```python
from build123d import *

# Parameters (mm, degrees)
SKETCH_1_R      = 1.5
SKETCH_1_R_2    = 0.5
SKETCH_1_W      = 23
SKETCH_1_H      = 12
EXTRUDE_1_DEPTH = 3


with BuildPart() as part:
    # 草图1 → 凸台-拉伸1 (new body)
    with BuildSketch(Plane(origin=(0, 0, 0), x_dir=(1, 0, 0), z_dir=(0, 1, 0))):
        Polygon((22.594315567, 25.84326654), (22.594315567, 28.84326654), (-7.405684433, 28.84326654), (-7.405684433, 25.84326654), (-10.405684433, 25.84326654), (-10.405684433, 28.84326654), (-40.405684433, 28.84326654), (-40.405684433, 25.84326654), (-43.405684433, 25.84326654), (-43.405684433, 28.84326654), (-44.905684433, 28.84326654), (-44.905684433, 10.84326654), (-43.405684433, 10.84326654), (-43.405684433, 13.84326654), (-40.405684433, 13.84326654), (-40.405684433, 10.84326654), (-10.405684433, 10.84326654), (-10.405684433, 14.84326654), (-7.405684433, 14.84326654), (-7.405684433, 10.84326654), (22.594315567, 10.84326654), (22.594315567, 13.84326654), (25.594315567, 13.84326654), (25.594315567, 10.84326654), (27.094315567, 10.84326654), (27.094315567, 28.84326654), (25.594315567, 28.84326654), (25.594315567, 25.84326654), align=None)
        with Locations(Location((-8.905684433, 19.84326654, 0), (0, 0, 270))):
            Circle(SKETCH_1_R, mode=Mode.SUBTRACT)
        with Locations(Location((-4.505684433, 19.84326654, 0), (0, 0, 270))):
            Circle(SKETCH_1_R_2, mode=Mode.SUBTRACT)
        with Locations(Location((-40.805684433, 19.84326654, 0), (0, 0, 270))):
            Circle(SKETCH_1_R_2, mode=Mode.SUBTRACT)
        with Locations(Location((-13.305684433, 19.84326654, 0), (0, 0, 270))):
            Circle(SKETCH_1_R_2, mode=Mode.SUBTRACT)
        with Locations(Location((22.994315567, 19.84326654, 0), (0, 0, 270))):
            Circle(SKETCH_1_R_2, mode=Mode.SUBTRACT)
        with Locations((9.094315567, 19.84326654)):
            Rectangle(SKETCH_1_W, SKETCH_1_H, mode=Mode.SUBTRACT)
        with Locations((-26.905684433, 19.84326654)):
            Rectangle(SKETCH_1_W, SKETCH_1_H, mode=Mode.SUBTRACT)
    extrude(amount=EXTRUDE_1_DEPTH)


solid = part.part
```
Work out the finished part from the listing and answer in its coordinate system (mm). A direction names the side the tool comes from. Give positions to 0.01 mm unless a question says otherwise; leave off trailing zeros. Loops run counter-clockwise (first coordinate to the right, second up) from the corner with the lowest first, then second, coordinate; pieces in that order, holes last. Notation, with made-up numbers: (-1.5, 24.25) -> (22.5, 24.25) arc R19 ccw to (22.5, 37.25) -> close; hole circle Ø11 at (-16.5, 14). An arc over 180 degrees is marked (long way). Put each result on its own line as item: value. Start each with the question number.
Item 1: Each of these flat-tipped pins is pushed along its axis until it touches: P1, Ø1.8, axis at x = -8.91, z = -19.84, coming from the +Y side; P2, Ø0.9, axis at x = 24.5, y = 1.5, coming from the +Z side. Where does it stop, or does it pass through?
Item 2: The part is cut by section C-C (z = -26.5). Give the vertices of the cut face in (x, y), then the cut area to 3 significant figures.
Item 3: Which of the six approach directions +Z, -Z, +X, -X, +Y, -Y give full straight-line access (tool end or side, diameter ignored) to faces 4 (the face through (-10.406, 1, -13)), 5 (the face through (-25, 1, -28.843)), 6 (the face through (-15.406, 1, -20)), 7 (the face through (-42, 1, -25.843))?
Item 4: The part is cut by section B-B (z = -16). Give the vertices of the cut face in (x, y), then the cut area to 3 significant figures.
Item 5: Find the intervals of material crossed by L1, parallel to X at y = 2.6, z = -17.5; L2, parallel to X at y = 1.65, z = -27; L3, parallel to X at y = 1.4, z = -14.75, in increasing order. Write a range as [from, to].
Item 6: The mould has two halves that part along X. Classify faces 1 (the face through (-9, 3, -22)), 2 (the face through (-44.906, 1, -20)), 3 (the face through (-42, 1, -13.843)): released by +X, released by -X, zero draft, split by the parting line, or undercut.
Item 7: The part is cut by section A-A (x = -30.5). Give the vertices of the cut face in (y, z).
Item 8: The part is cut by section D-D (y = 0.75). State how many separate pieces and enclosed holes the cut face has, then the cut area to 3 significant figures.
Answers below:
1. P1: through
1. P2: z = -13.84
2. outline: (-44.91, 0) -> (-43.41, 0) -> (-43.41, 3) -> (-44.91, 3) -> close; (-40.41, 0) -> (-10.41, 0) -> (-10.41, 3) -> (-40.41, 3) -> close; (-7.41, 0) -> (22.59, 0) -> (22.59, 3) -> (-7.41, 3) -> close; (25.59, 0) -> (27.09, 0) -> (27.09, 3) -> (25.59, 3) -> close
2. area: 189 mm2
3. face 4: +Z, +Y, -Y
3. face 5: -Z, +X, -X, +Y, -Y
3. face 6: +Y, -Y
3. face 7: -Z, +Y, -Y
4. outline: (-44.91, 0) -> (-38.41, 0) -> (-38.41, 3) -> (-44.91, 3) -> close; (-15.41, 0) -> (-2.41, 0) -> (-2.41, 3) -> (-15.41, 3) -> close; (20.59, 0) -> (27.09, 0) -> (27.09, 3) -> (20.59, 3) -> close
4. area: 78.0 mm2
5. L1: [-44.91, -38.41], [-15.41, -2.41], [20.59, 27.09]
5. L2: [-44.91, -43.41], [-40.41, -10.41], [-7.41, 22.59], [25.59, 27.09]
5. L3: [-44.91, -38.41], [-15.41, -10.41], [-7.41, -2.41], [20.59, 27.09]
6. face 1: zero draft
6. face 2: released by -X
6. face 3: undercut
7. outline: (0, -28.84) -> (3, -28.84) -> (3, -25.84) -> (0, -25.84) -> close; (0, -13.84) -> (3, -13.84) -> (3, -10.84) -> (0, -10.84) -> close
8. separate pieces: 1
8. enclosed holes: 7
8. area: 677 mm2
